```python
from build123d import *

# Parameters (mm, degrees)
SKETCH1_R               = 18.1
BOSS_EXTRUDE1_DEPTH     = 33.3
SKETCH2_R               = 18.5
BOSS_EXTRUDE2_DEPTH     = 35.3568
SKETCH3_R               = 6
BOSS_EXTRUDE3_DEPTH     = 5
SKETCH4_R               = 3
BOSS_EXTRUDE4_DEPTH     = 15
CUT_EXTRUDE1_DEPTH      = 93.436617129
CUT_EXTRUDE1_DEPTH_BACK = 93.436617129
SKETCH5_W               = 0.5
SKETCH5_H               = 14
SKETCH6_R               = 1.5
CUT_EXTRUDE2_DEPTH      = 10
CIRPATTERN1_COUNT       = 6


with BuildPart() as part:
    # Sketch1 → Boss-Extrude1 (new body)
    with BuildSketch(Plane(origin=(0, 0, 0), x_dir=(1, 0, 0), z_dir=(0, 1, 0))):
        with Locations(Location((0, 0, 0), (0, 0, 270))):
            Circle(SKETCH1_R)
    extrude(amount=BOSS_EXTRUDE1_DEPTH)

    # Sketch2 → Boss-Extrude2 (add)
    with BuildSketch(Plane(origin=(0, 33.3, 0), x_dir=(1, 0, 0), z_dir=(0, 1, 0))):
        with Locations(Location((0, 0, 0), (0, 0, 270))):
            Circle(SKETCH2_R)
    extrude(amount=BOSS_EXTRUDE2_DEPTH)

    # Sketch3 → Boss-Extrude3 (add)
    with BuildSketch(Plane(origin=(0, 68.6568, 0), x_dir=(1, 0, 0), z_dir=(0, 1, 0))):
        with Locations(Location((0, 0, 0), (0, 0, 270))):
            Circle(SKETCH3_R)
    extrude(amount=BOSS_EXTRUDE3_DEPTH)

    # Sketch4 → Boss-Extrude4 (add)
    with BuildSketch(Plane(origin=(0, 73.6568, 0), x_dir=(1, 0, 0), z_dir=(0, 1, 0))):
        with Locations(Location((0, 0, 0), (0, 0, 270))):
            Circle(SKETCH4_R)
    extrude(amount=BOSS_EXTRUDE4_DEPTH)

    # Sketch5 → Cut-Extrude1 (cut, two sides: drawn at the far end of the back side and taken through both)
    with BuildSketch(Plane.XY.offset(-CUT_EXTRUDE1_DEPTH_BACK)):
        with Locations((2.75, 81.6568)):
            Rectangle(SKETCH5_W, SKETCH5_H)
    extrude(amount=CUT_EXTRUDE1_DEPTH + CUT_EXTRUDE1_DEPTH_BACK, mode=Mode.SUBTRACT)

    # Sketch6 → Cut-Extrude2 (cut)
    with BuildSketch(Plane(origin=(0, 68.6568, 0), x_dir=(1, 0, 0), z_dir=(0, 1, 0))):
        with Locations(Location((0, 15.5, 0), (0, 0, 270))):
            Circle(SKETCH6_R)
    cut_extrude2 = extrude(amount=-CUT_EXTRUDE2_DEPTH, mode=Mode.SUBTRACT)

    # CirPattern1: Cut-Extrude2 ×6 about axis
    cirpattern1_axis = Axis((0, 0, 0), (0, 1, 0))
    for i in range(1, CIRPATTERN1_COUNT):
        add(cut_extrude2.rotate(cirpattern1_axis, i * 360 / CIRPATTERN1_COUNT), mode=Mode.SUBTRACT)


solid = part.part
```
Read the model definition and answer for the solid it produces. Units are mm, in the model's axes. A direction names the side the tool comes from. Give positions to 0.01 mm unless a question says otherwise; leave off trailing zeros. Write each loop counter-clockwise with the first axis right and the second up, starting at its lowest first coordinate (ties: lowest second). Pieces come first, ordered by that corner, then holes. Notation, with made-up numbers: (68, -7.5) -> (81, -7.5) arc R18 ccw to (81, 18.5) -> close; hole circle Ø8 at (35.5, 67.5). An arc over 180 degrees is marked (long way). Answer in a Markdown table with one row per item.
1) Determine the mould class of faces 1 (the cylindrical face through (-14.754, 63.727, 8.442)), 2 (the flat face through (2.5, 82, 0)), 3 (the cylindrical face through (-7.086, 50.731, 17.089)) for opening direction Z: released by +Z, released by -Z, zero draft, split by the parting line, or undercut.
Results list:
| item | result |
|---|---|
| face 1 | undercut |
| face 2 | zero draft |
| face 3 | split by the parting line |
2) Section B-B on z = 0 is taken. Give the vertices of the cut face in (x, y).
Results list:
| item | result |
|---|---|
| outline | (-18.5, 33.3) -> (-18.1, 33.3) -> (-18.1, 0) -> (18.1, 0) -> (18.1, 33.3) -> (18.5, 33.3) -> (18.5, 68.66) -> (6, 68.66) -> (6, 73.66) -> (3, 73.66) -> (3, 74.66) -> (2.5, 74.66) -> (2.5, 88.66) -> (-3, 88.66) -> (-3, 73.66) -> (-6, 73.66) -> (-6, 68.66) -> (-18.5, 68.66) -> close |
3) A tool of negligible diameter and unlimited length cuts with its end or side. For faces 4 (the flat face through (-13.6, 33.3, 12.2)), 5 (the flat face through (0, 88.657, 0)), 6 (the flat face through (0, 58.657, -16)), from which of +Z, -Z, +X, -X, +Y, -Y can it reach the whole face along a straight path? Write none if from no direction.
Results list:
| item | result |
|---|---|
| face 4 | -Y |
| face 5 | +Z, -Z, +X, -X, +Y |
| face 6 | +Y |
4) Section A-A on x = 0 is taken. Give the vertices of the cut face in (y, z).
Results list:
| item | result |
|---|---|
| outline | (0, -18.1) -> (33.3, -18.1) -> (33.3, -18.5) -> (68.66, -18.5) -> (68.66, -17) -> (58.66, -17) -> (58.66, -14) -> (68.66, -14) -> (68.66, -6) -> (73.66, -6) -> (73.66, -3) -> (88.66, -3) -> (88.66, 3) -> (73.66, 3) -> (73.66, 6) -> (68.66, 6) -> (68.66, 14) -> (58.66, 14) -> (58.66, 17) -> (68.66, 17) -> (68.66, 18.5) -> (33.3, 18.5) -> (33.3, 18.1) -> (0, 18.1) -> close |
5) Section D-D on z = -13 is taken. Give the vertices of the cut face in (x, y), plus the area to 3 significant figures.
Results list:
| item | result |
|---|---|
| outline | (-13.16, 33.3) -> (-12.59, 33.3) -> (-12.59, 0) -> (12.59, 0) -> (12.59, 33.3) -> (13.16, 33.3) -> (13.16, 68.66) -> (-13.16, 68.66) -> close |
| area | 1,770 mm^2 |
6) Straight lines are drawn through the part: line 1 (X direction, y = 61, z = -9); line 2 (X direction, y = 66, z = 7.75); line 3 (Y direction, x = -1, z = -5.5). For each, find the intervals that lie inside material, in ascending order. Write a range as [from, to].
Results list:
| item | result |
|---|---|
| line 1 | [-16.16, -14.25], [-12.59, 12.59], [14.25, 16.16] |
| line 2 | [-16.8, -14.92], [-11.92, 11.92], [14.92, 16.8] |
| line 3 | [0, 73.66] |
7) Each of these flat-tipped pins is pushed along its axis until it touches: pin 1 Ø1 at (x, y) = (11.5, 49) entering from -Z; pin 2 Ø2 at (x, z) = (11.5, 5) entering from -Y; pin 3 Ø2.5 at (x, z) = (-13.42, 7.75) entering from +Y; pin 4 Ø1 at (y, z) = (80, 0.5) entering from +X. Where does it stop, or does it pass through?
Results list:
| item | result |
|---|---|
| pin 1 | z = -14.87 |
| pin 2 | y = 0 |
| pin 3 | y = 58.66 |
| pin 4 | x = 2.5 |
8) Section C-C on y = 36 is taken. Give the vertices of the cut face in (x, z).
Results list:
| item | result |
|---|---|
| outline | circle Ø37 at (0, 0) |
